```python
from build123d import *

# Parameters (mm, degrees)
SKETCH1_R           = 21.5
SKETCH1_R_2         = 1.25
SKETCH1_R_3         = 7.5
BOSS_EXTRUDE1_DEPTH = 3
SKETCH1_3_R         = 1.25
BOSS_EXTRUDE2_DEPTH = 3
BOSS_EXTRUDE6_DEPTH = 20


with BuildPart() as part:
    # Sketch1 → Boss-Extrude1 (new body)
    with BuildSketch(Plane.XY):
        Circle(SKETCH1_R)
        with Locations((-13.435028843, 13.435028843)):
            Circle(SKETCH1_R_2, mode=Mode.SUBTRACT)
        with Locations((13.435028843, 13.435028843)):
            Circle(SKETCH1_R_2, mode=Mode.SUBTRACT)
        with Locations((13.435028843, -13.435028843)):
            Circle(SKETCH1_R_2, mode=Mode.SUBTRACT)
        with Locations((-13.435028843, -13.435028843)):
            Circle(SKETCH1_R_2, mode=Mode.SUBTRACT)
        with Locations((-12.85, 0)):
            Circle(SKETCH1_R_2, mode=Mode.SUBTRACT)
        with Locations((-6.425, 11.128426439)):
            Circle(SKETCH1_R_2, mode=Mode.SUBTRACT)
        with Locations((6.425, 11.128426439)):
            Circle(SKETCH1_R_2, mode=Mode.SUBTRACT)
        with Locations((12.85, 0)):
            Circle(SKETCH1_R_2, mode=Mode.SUBTRACT)
        with Locations((6.425, -11.128426439)):
            Circle(SKETCH1_R_2, mode=Mode.SUBTRACT)
        with Locations((-6.425, -11.128426439)):
            Circle(SKETCH1_R_2, mode=Mode.SUBTRACT)
        Circle(SKETCH1_R_3, mode=Mode.SUBTRACT)
    extrude(amount=BOSS_EXTRUDE1_DEPTH)

    # Sketch1_3 → Boss-Extrude2 (add)
    with BuildSketch(Plane.XY):
        with BuildLine():
            ThreePointArc((-15.244012286, 6.314276634), (-11.66726189, 11.66726189), (-6.314276634, 15.244012286))
            Line((-6.314276634, 15.244012286), (-8.227693796, 19.863409949))
            ThreePointArc((-8.227693796, 19.863409949), (-15.202795796, 15.202795796), (-19.863409949, 8.227693796))
            Line((-19.863409949, 8.227693796), (-15.244012286, 6.314276634))
        make_face()
        with Locations((-13.435028843, 13.435028843)):
            Circle(SKETCH1_3_R, mode=Mode.SUBTRACT)
        with BuildLine():
            ThreePointArc((19.863409949, 8.227693796), (15.202795796, 15.202795796), (8.227693796, 19.863409949))
            Line((8.227693796, 19.863409949), (6.314276634, 15.244012286))
            ThreePointArc((6.314276634, 15.244012286), (11.66726189, 11.66726189), (15.244012286, 6.314276634))
            Line((15.244012286, 6.314276634), (19.863409949, 8.227693796))
        make_face()
        with Locations((13.435028843, 13.435028843)):
            Circle(SKETCH1_3_R, mode=Mode.SUBTRACT)
        with BuildLine():
            ThreePointArc((-6.314276634, -15.244012286), (-11.66726189, -11.66726189), (-15.244012286, -6.314276634))
            Line((-15.244012286, -6.314276634), (-19.863409949, -8.227693796))
            ThreePointArc((-19.863409949, -8.227693796), (-15.202795796, -15.202795796), (-8.227693796, -19.863409949))
            Line((-8.227693796, -19.863409949), (-6.314276634, -15.244012286))
        make_face()
        with Locations((-13.435028843, -13.435028843)):
            Circle(SKETCH1_3_R, mode=Mode.SUBTRACT)
        with BuildLine():
            ThreePointArc((15.244012286, -6.314276634), (11.66726189, -11.66726189), (6.314276634, -15.244012286))
            Line((6.314276634, -15.244012286), (8.227693796, -19.863409949))
            ThreePointArc((8.227693796, -19.863409949), (15.202795796, -15.202795796), (19.863409949, -8.227693796))
            Line((19.863409949, -8.227693796), (15.244012286, -6.314276634))
        make_face()
        with Locations((13.435028843, -13.435028843)):
            Circle(SKETCH1_3_R, mode=Mode.SUBTRACT)
    extrude(amount=-BOSS_EXTRUDE2_DEPTH)

    # Sketch7 → Boss-Extrude6 (add)
    with BuildSketch(Plane.XY.offset(3)):
        with BuildLine():
            ThreePointArc((10.75, 18.619546181), (0, 21.5), (-10.75, 18.619546181))
            Line((-10.75, 18.619546181), (-8.25, 14.289419162))
            ThreePointArc((-8.25, 14.289419162), (0, 16.5), (8.25, 14.289419162))
            Line((8.25, 14.289419162), (10.75, 18.619546181))
        make_face()
        with BuildLine():
            ThreePointArc((21.5, 0), (20.767405265, 5.56460947), (18.619546181, 10.75))
            Line((18.619546181, 10.75), (14.289419162, 8.25))
            ThreePointArc((14.289419162, 8.25), (16.5, 0), (14.289419162, -8.25))
            Line((14.289419162, -8.25), (18.619546181, -10.75))
            ThreePointArc((18.619546181, -10.75), (20.767405265, -5.56460947), (21.5, 0))
        make_face()
        with BuildLine():
            Line((-8.25, -14.289419162), (-10.75, -18.619546181))
            ThreePointArc((-10.75, -18.619546181), (0, -21.5), (10.75, -18.619546181))
            Line((10.75, -18.619546181), (8.25, -14.289419162))
            ThreePointArc((8.25, -14.289419162), (0, -16.5), (-8.25, -14.289419162))
        make_face()
        with BuildLine():
            ThreePointArc((-14.289419162, -8.25), (-16.5, 0), (-14.289419162, 8.25))
            Line((-14.289419162, 8.25), (-18.619546181, 10.75))
            ThreePointArc((-18.619546181, 10.75), (-21.5, 0), (-18.619546181, -10.75))
            Line((-18.619546181, -10.75), (-14.289419162, -8.25))
        make_face()
    extrude(amount=BOSS_EXTRUDE6_DEPTH)


solid = part.part
```
The listing builds one solid part. Answer for the finished solid, in the listing's coordinates (mm). A direction names the side the tool comes from. Coordinates: 2 decimals unless noted, no trailing zeros. Loops run counter-clockwise (first coordinate to the right, second up) from the corner with the lowest first, then second, coordinate; pieces in that order, holes last. Notation, with made-up numbers: M -20,48 L 16,48 A30 cw 16,82 Z; hole C 28,-10.75 d9. An arc over 180 degrees is marked long. Answer as CSV lines item,"result". Start each with the question number.
(1) The part is cut by section C-C (x = 12.85). Give the vertices of the cut face in (y, z), and give its area (3 significant figures).
(2) The part is cut by section A-A (z = 20). Give the vertices of the cut face in (x, y).
(3) The mould has two halves that part along X. Classify faces 1 (the flat face through (-18, 0, 23)), 2 (the flat face through (17.586, -7.284, -1.479)), 3 (the cylindrical face through (-11.731, 11.603, -1.479)): pulls with the +X half, pulls with the -X half, needs draft (parallel to the pull), parting line crosses it, or undercut.
(4) The part is cut by section D-D (z = 1). State how many separate pieces and enclosed holes the cut face has, and give its area (3 significant figures).
(5) Find the intervals of material crossed by L1, parallel to Y at x = 12.85, z = 1.7; L2, parallel to Y at x = -14, z = -1.25; L3, parallel to X at y = -10, z = 0.25, in increasing order. Write a range as [from, to].
(6) Given pin 1 (3 mm diameter, centred on x = 6.42, y = -11.13, fed in from -Z); pin 2 (1.5 mm diameter, centred on x = 6.5, z = 18, fed in from -Y); pin 3 (2 mm diameter, centred on x = -6.42, y = 11.13, fed in from -Z); pin 4 (1 mm diameter, centred on y = 16, z = 7, fed in from +X), each flat-ended and moving along its own axis, determine where each tip first touches the part or whether it passes through.
(7) The part is cut by section B-B (x = 0). Give the vertices of the cut face in (y, z), and give its area (3 significant figures).
(8) For faces 4 (the flat face through (16.42, -9.48, 12.86)), 5 (the cylindrical face through (-0.1, 16.5, 12.9)), 6 (the flat face through (-10, 0, 0)), 7 (the flat face through (-9.48, -16.42, 12.86)), 8 (the flat face through (-7.258, 17.521, -1.479)), determine the directions among +Z, -Z, +X, -X, +Y, -Y from which every point of the face is accessible in a straight line to the end or side of a thin tool.
Determined:
1,outline,"M -17.24,-3 L -14.54,-3 L -14.54,3 L -17.24,3 Z; M -12.33,-3 L -10.35,-3 L -10.35,0 L -1.25,0 L -1.25,3 L -12.33,3 Z; M 1.25,0 L 10.35,0 L 10.35,-3 L 12.33,-3 L 12.33,3 L 1.25,3 Z; M 14.54,-3 L 17.24,-3 L 17.24,3 L 14.54,3 Z"
1,area,"111 mm2"
2,outline,"M -18.62,-10.75 L -14.29,-8.25 A16.5 cw -14.29,8.25 L -18.62,10.75 A21.5 ccw Z; M -10.75,-18.62 A21.5 ccw 10.75,-18.62 L 8.25,-14.29 A16.5 cw -8.25,-14.29 Z; M -10.75,18.62 L -8.25,14.29 A16.5 cw 8.25,14.29 L 10.75,18.62 A21.5 ccw Z; M 14.29,-8.25 L 18.62,-10.75 A21.5 ccw 18.62,10.75 L 14.29,8.25 A16.5 cw Z"
3,face 1,"needs draft"
3,face 2,"pulls with the +X half"
3,face 3,"undercut"
4,separate pieces,"1"
4,enclosed holes,"11"
4,area,"1,230 mm2"
5,L1,"[-17.24, -14.54], [-12.33, -1.25], [1.25, 12.33], [14.54, 17.24]"
5,L2,"[-16.32, -14.55], [-12.32, -8.73], [8.73, 12.32], [14.55, 16.32]"
5,L3,"[-19.03, -6.96], [-5.89, 5.89], [6.96, 19.03]"
6,pin 1,"z = 0"
6,pin 2,"y = -20.72"
6,pin 3,"through"
6,pin 4,"x = 9.53"
7,outline,"M -21.5,0 L -7.5,0 L -7.5,3 L -16.5,3 L -16.5,23 L -21.5,23 Z; M 7.5,0 L 21.5,0 L 21.5,23 L 16.5,23 L 16.5,3 L 7.5,3 Z"
7,area,"284 mm2"
8,face 4,"+Z, -Y"
8,face 5,"+Z"
8,face 6,"-Z"
8,face 7,"+Z, -X"
8,face 8,"-Z, +Y"
